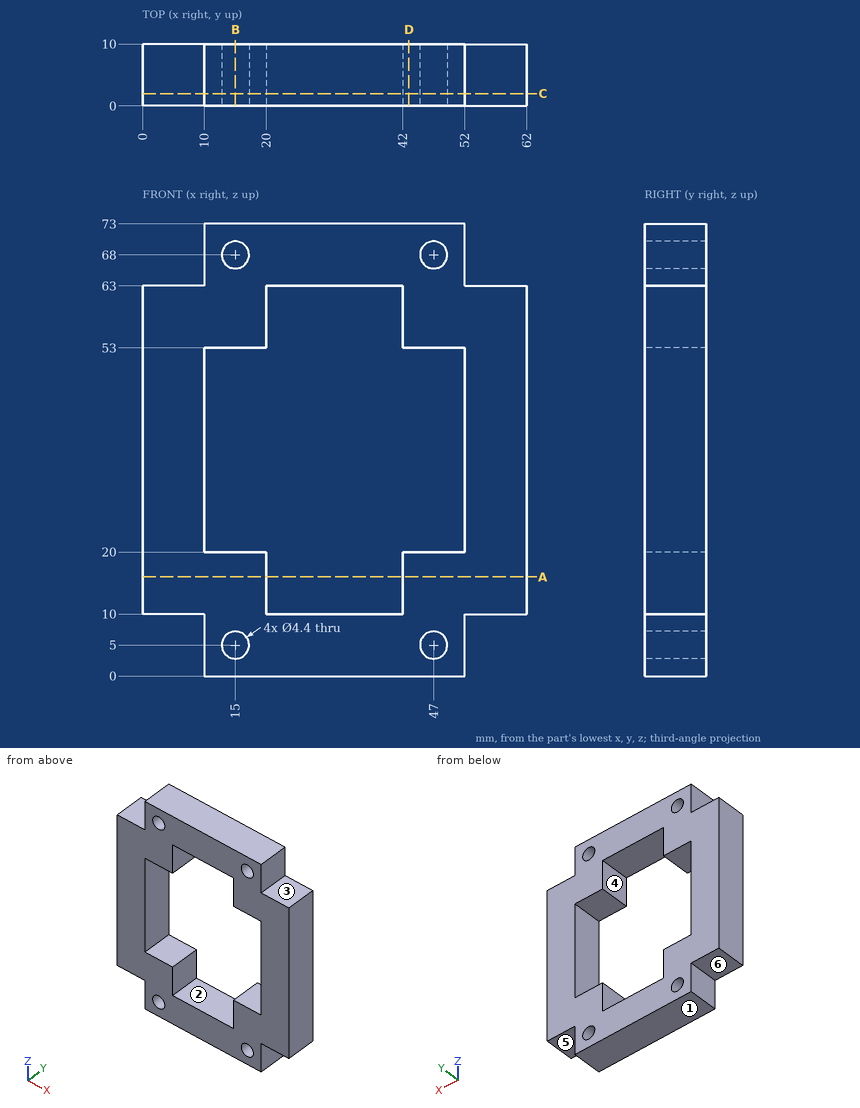
Part print with two shaded views. Sizes in mm from the minimum x, y, z corner. A direction names the side the tool comes from. Coordinates: 2 decimals unless noted, no trailing zeros. Write each loop counter-clockwise with the first axis right and the second up, starting at its lowest first coordinate (ties: lowest second). Pieces come first, ordered by that corner, then holes.
(1) Drill centre lines: line 1 (Z direction, x = 15, y = 3.75); line 2 (X direction, y = 5, z = 5); line 3 (X direction, y = 4.75, z = 46). Where is each one in solid material? Low to high.
(2) 3-axis set-ups, long thin cutter, end or side, ignore diameter. For the marked faces 4, 5 and 6: which of +Z, -Z, +X, -X, +Y, -Y reach the whole face in a straight line?
(3) Pin check, flat tips, straight feed: pin 1 Ø3 at (x, z) = (37.5, 60) entering from +Y; pin 2 Ø5 at (y, z) = (7.5, 67) entering from -X; pin 3 Ø5 at (x, y) = (59.5, 3) entering from +Z; pin 4 Ø5 at (x, y) = (59, 6.5) entering from -Z. Stop position of each tip, or through.
(4) Cut at A-A on z = 16. List the corners of the cut face in (x, y), and give its area (3 significant figures).
(5) Cut at C-C on y = 2. List the corners of the cut face in (x, z).
(6) Cut at B-B on x = 15. List the corners of the cut face in (y, z).
(7) Mould opens along Z. For the marked faces 1, 2 and 3 say: pulls with the +Z half, pulls with the -Z half, needs draft (parallel to the pull), parting line crosses it, or undercut.
(8) Cut at D-D on x = 43. List the corners of the cut face in (y, z), and give its area (3 significant figures).
Working result:
1. line 1: z = 0 to 2.8, 7.2 to 20, 53 to 65.8, 70.2 to 73
1. line 2: x = 10 to 12.8, 17.2 to 44.8, 49.2 to 52
1. line 3: x = 0 to 10, 52 to 62
2. face 4: +Y, -Y
2. face 5: -Z, +X, +Y, -Y
2. face 6: -Z, -X, +Y, -Y
3. pin 1: passes through
3. pin 2: stops at x = 10
3. pin 3: stops at z = 63
3. pin 4: stops at z = 10
4. outline: (0, 0) - (20, 0) - (20, 10) - (0, 10) - close; (42, 0) - (62, 0) - (62, 10) - (42, 10) - close
4. area: 400 mm2
5. outline: (0, 10) - (10, 10) - (10, 0) - (52, 0) - (52, 10) - (62, 10) - (62, 63) - (52, 63) - (52, 73) - (10, 73) - (10, 63) - (0, 63) - close; hole (10, 20) - (20, 20) - (20, 10) - (42, 10) - (42, 20) - (52, 20) - (52, 53) - (42, 53) - (42, 63) - (20, 63) - (20, 53) - (10, 53) - close; hole circle Ø4.4 at (15, 5); hole circle Ø4.4 at (15, 68); hole circle Ø4.4 at (47, 5); hole circle Ø4.4 at (47, 68)
6. outline: (0, 0) - (10, 0) - (10, 2.8) - (0, 2.8) - close; (0, 7.2) - (10, 7.2) - (10, 20) - (0, 20) - close; (0, 53) - (10, 53) - (10, 65.8) - (0, 65.8) - close; (0, 70.2) - (10, 70.2) - (10, 73) - (0, 73) - close
7. face 1: pulls with the -Z half
7. face 2: undercut
7. face 3: pulls with the +Z half
8. outline: (0, 0) - (10, 0) - (10, 20) - (0, 20) - close; (0, 53) - (10, 53) - (10, 73) - (0, 73) - close
8. area: 400 mm2
